Geometry: see drawing. Coordinates: mm, zero at the bounding-box minimum. Round coordinates to 2 decimals unless told otherwise and drop trailing zeros. Order: outer loops, then holes, each group sorted by start corner. A loop starts at its lowest first (then second) coordinate and runs counter-clockwise, first axis right, second up. Notation, with made-up numbers: (-27.5, -2.75) -> (23.5, -2.75) arc R6 ccw to (23.5, 7.25) -> close; hole circle Ø2 at (-24.75, 11.5). An arc over 180 degrees is marked (long way). Write item = value, one per line. Start each with the question number.
(1) Contact query for flat-ended pins moving along their axis: pin 1 Ø0.8 at (y, z) = (1, 66.5) entering from +X; pin 2 Ø1 at (y, z) = (5, 16.5) entering from +X; pin 3 Ø1.9 at (x, z) = (62.639, 2.377) entering from +Y; pin 4 Ø1.7 at (x, y) = (30.5, 5.5) entering from +Z. Output: stop coordinate, or through.
(2) Cut plane A-A on x = 34.5. Return the cut outline in (y, z) (1 decimal).
(3) Cut plane C-C on x = 23. Return the cut outline in (y, z) (1 decimal), then the cut area to 3 significant figures.
(4) Ray query, line 1 (X direction, y = 4.25, z = 38.5); line 2 (X direction, y = 1, z = 3) (1 decimal); line 3 (Z direction, x = 14, y = 5). Return the intervals inside material, ascending.
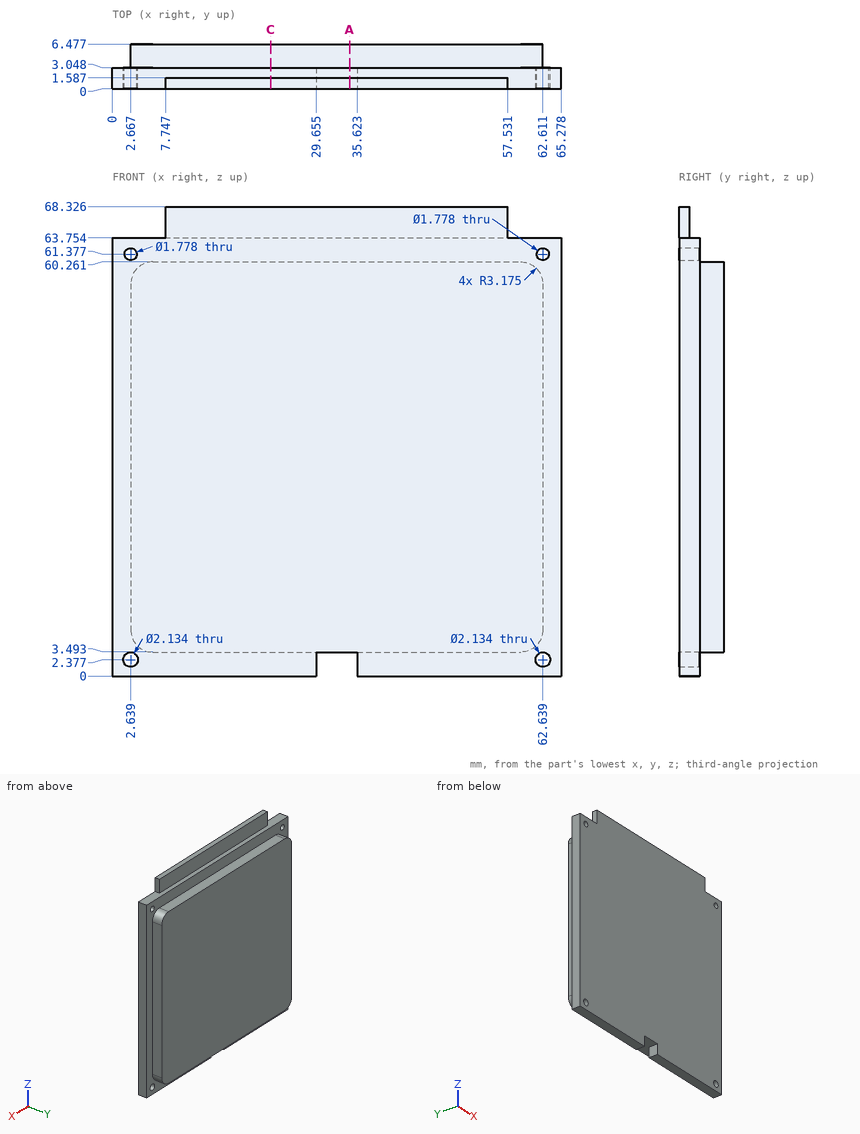
Evaluation:
q1.pin_1 = 57.53
q1.pin_2 = 62.61
q1.pin_3 = through
q1.pin_4 = 60.26
q2.outline = (0, 3.5) -> (6.5, 3.5) -> (6.5, 60.3) -> (3, 60.3) -> (3, 63.8) -> (1.6, 63.8) -> (1.6, 68.3) -> (0, 68.3) -> close
q3.outline = (0, 0) -> (3, 0) -> (3, 3.5) -> (6.5, 3.5) -> (6.5, 60.3) -> (3, 60.3) -> (3, 63.8) -> (1.6, 63.8) -> (1.6, 68.3) -> (0, 68.3) -> close
q3.area = 396 mm^2
q4.line_1 = 2.67 to 62.61
q4.line_2 = 0 to 1.8, 3.5 to 29.7, 35.6 to 61.8, 63.5 to 65.3
q4.line_3 = 3.49 to 60.26
